Autodesk Inventor part; units mm, degrees
ref_plane "YZ Plane" through (0, 0, 0) normal (1, 0, 0) x (0, 1, 0)
ref_plane "XZ Plane" through (0, 0, 0) normal (0, 1, 0) x (-1, 0, 0)
ref_plane "XY Plane" through (0, 0, 0) normal (0, 0, 1) x (1, 0, 0)
sketch "スケッチ1" plane through (0, 0, 0) normal (0, 0, 1) x (1, 0, 0)
  line L0 (-29, -29) -> (29, -29)
  line L1 (29, -29) -> (29, 29)
  line L2 (29, 29) -> (-29, 29)
  line L3 (-29, 29) -> (-29, -29)
  line L4 (-29, -29) -> (29, 29) construction
  line L5 (29, -29) -> (-29, 29) construction
  point P0 (0, 0)
  dimension "d0" = 58
  dimension "d1" = 58
extrude "押し出し1" add sketch "スケッチ1" along normal blind 6
fillet "フィレット1" radius 5 4 edges at (-29, 29, 3) (29, 29, 3) (29, -29, 3) (-29, -29, 3)
sketch "スケッチ4" plane through (0, 0, 6) normal (0, 0, 1) x (1, 0, 0)
  arc A0 (-29, -24) -> (-24, -29) centre (-24, -24) ccw
  line L0 (-24, -29) -> (24, -29)
  arc A1 (24, -29) -> (29, -24) centre (24, -24) ccw
  line L1 (29, -24) -> (29, 24)
  arc A2 (29, 24) -> (24, 29) centre (24, 24) ccw
  line L2 (24, 29) -> (-24, 29)
  arc A3 (-24, 29) -> (-29, 24) centre (-24, 24) ccw
  line L3 (-29, 24) -> (-29, -24)
  line L4 (-27, -27) -> (27, -27)
  line L5 (27, -27) -> (27, 27)
  line L6 (27, 27) -> (-27, 27)
  line L7 (-27, 27) -> (-27, -27)
  line L8 (-27, -27) -> (27, 27) construction
  line L9 (27, -27) -> (-27, 27) construction
  line L10 (-24, -24) -> (24, -24) construction
  line L11 (24, -24) -> (24, 24) construction
  line L12 (24, 24) -> (-24, 24) construction
  line L13 (-24, 24) -> (-24, -24) construction
  line L14 (-24, -24) -> (24, 24) construction
  line L15 (24, -24) -> (-24, 24) construction
  line L16 (24, 29) -> (-24, 29)
  circle A4 centre (-24, 24) radius 5
  circle A5 centre (24, 24) radius 5
  arc A6 (24, -29) -> (29, -24) centre (24, -24) ccw
  circle A7 centre (24, -24) radius 5
  line L17 (-24, -29) -> (24, -29)
  circle A8 centre (-24, -24) radius 5
  line L18 (-29, 29) -> (-19, 29)
  line L19 (-19, 29) -> (-19, 19)
  line L20 (-19, 19) -> (-29, 19)
  line L21 (-29, 19) -> (-29, 29)
  line L22 (-29, 29) -> (-19, 19) construction
  line L23 (-19, 29) -> (-29, 19) construction
  line L24 (29, 29) -> (19, 29)
  line L25 (19, 29) -> (19, 19)
  line L26 (19, 19) -> (29, 19)
  line L27 (29, 19) -> (29, 29)
  line L28 (29, 29) -> (19, 19) construction
  line L29 (19, 29) -> (29, 19) construction
  line L30 (29, -29) -> (19, -29)
  line L31 (19, -29) -> (19, -19)
  line L32 (19, -19) -> (29, -19)
  line L33 (29, -19) -> (29, -29)
  line L34 (29, -29) -> (19, -19) construction
  line L35 (19, -29) -> (29, -19) construction
  line L36 (-29, -29) -> (-19, -29)
  line L37 (-19, -29) -> (-19, -19)
  line L38 (-19, -19) -> (-29, -19)
  line L39 (-29, -19) -> (-29, -29)
  line L40 (-29, -29) -> (-19, -19) construction
  line L41 (-19, -29) -> (-29, -19) construction
  point P0 (0, 0)
  point P1 (-20, -27)
  point P2 (20, -27)
  point P3 (27, -20)
  point P4 (27, 20)
  point P5 (20, 27)
  point P6 (-20, 27)
  point P7 (-27, 20)
  point P8 (-27, -20)
  point P9 (-19, -24)
  point P10 (-19, -27)
  point P11 (19, -27)
  point P12 (19, -24)
  point P13 (24, -19)
  point P14 (27, -19)
  point P15 (27, 19)
  point P16 (24, 19)
  point P17 (19, 24)
  point P18 (19, 27)
  point P19 (-19, 27)
  point P20 (-19, 24)
  point P21 (-24, 19)
  point P22 (-27, 19)
  point P23 (-27, -19)
  point P24 (-24, -19)
  dimension "d77" = 54
  dimension "d78" = 54
  dimension "d79" = 48
  dimension "d80" = 48
  dimension "d81" = 10
  dimension "d82" = 10
  dimension "d83" = 10
  dimension "d84" = 10
  dimension "d85" = 10
  dimension "d86" = 10
  dimension "d87" = 10
  dimension "d88" = 10
  dimension "d89" = 10
  dimension "d90" = 10
  dimension "d91" = 10
  dimension "d92" = 10
extrude "押し出し2" cut sketch "スケッチ4" against normal blind 4 contours L7 L20 L19 L6 L25 L26 L5 L32 L31 L4 L37 L38
sketch "スケッチ5" plane through (0, 0, 2) normal (0, 0, 1) x (1, 0, 0)
  circle A0 centre (0, 0) radius 16
  point P0 (-11.3137, 11.3137)
  point P1 (-11.3137, -11.3137)
  point P2 (11.3137, -11.3137)
  point P3 (11.3137, 11.3137)
  dimension "d18" = 32
  dimension "d21" = 360
  dimension "d58" = 0
hole "穴2" at (-11.3137, 11.3137, 2) at (-11.3137, -11.3137, 2) at (11.3137, -11.3137, 2) at (11.3137, 11.3137, 2) direction (0, 0, -1) diameter 4.5 depth 11.8 tip angle 118 counterbore diameter 8 counterbore depth 4
sketch "スケッチ6" plane through (0, 0, 2) normal (0, 0, 1) x (1, 0, 0)
  circle A0 centre (0, 0) radius 15
  point P0 (0, 15)
  point P1 (-15, 0)
  point P2 (0, -15)
  point P3 (15, 0)
  dimension "d30" = 30
  dimension "d33" = 360
  dimension "d59" = 0
hole "穴3" at (15, 0, 2) at (0, 15, 2) at (-15, 0, 2) direction (0, 0, -1) diameter 3.4 depth 11.8 tip angle 118
fillet "フィレット5" radius 3 8 edges at (-27, 19, 4) (-19, 27, 4) (19, 27, 4) (27, 19, 4) (27, -19, 4) (19, -27, 4) (-19, -27, 4) (-27, -19, 4)
sketch "スケッチ7" plane through (0, 0, 2) normal (0, 0, 1) x (1, 0, 0)
  circle A0 centre (0, 0) radius 10
  dimension "d42" = 20
extrude "押し出し3" cut sketch "スケッチ7" against normal through all
sketch "スケッチ8" plane through (0, 0, 6) normal (0, 0, 1) x (1, 0, 0)
  line L0 (24, -24) -> (-24, -24)
  line L1 (-24, -24) -> (-24, 24)
  line L2 (-24, 24) -> (24, 24)
  line L3 (24, 24) -> (24, -24)
  line L4 (24, -24) -> (-24, 24) construction
  line L5 (-24, -24) -> (24, 24) construction
  point P0 (0, 0)
  dimension "d45" = 48
  dimension "d46" = 48
hole "穴4" at (-24, 24, 6) at (-24, -24, 6) at (24, -24, 6) at (24, 24, 6) direction (0, 0, -1) diameter 3.4 depth 6 tip angle 118
sketch "スケッチ9" plane through (0, 0, 6) normal (0, 0, 1) x (1, 0, 0)
  line L0 (-20, -29) -> (20, -29)
  line L1 (20, -29) -> (20, -5)
  line L2 (20, -5) -> (-20, -5)
  line L3 (-20, -5) -> (-20, -29)
  line L4 (-20, -29) -> (20, -5) construction
  line L5 (20, -29) -> (-20, -5) construction
  line L6 (-24, -29) -> (24, -29)
  circle A0 centre (11.3137, -11.3137) radius 4
  line L7 (10, 5) -> (-10, 5)
  line L8 (-10, 5) -> (-10, -5)
  line L9 (-10, -5) -> (10, -5)
  line L10 (10, -5) -> (10, 5)
  line L11 (10, 5) -> (-10, -5) construction
  line L12 (-10, 5) -> (10, -5) construction
  circle A1 centre (0, 0) radius 10
  line L13 (-10, 0) -> (10, 0)
  point P0 (0, -17)
  point P1 (0, -17)
  point P2 (8.6603, -5)
  point P3 (-8.6603, -5)
  point P4 (-15, 0)
  dimension "d54" = 40
  dimension "d64" = 5
extrude "押し出し4" cut sketch "スケッチ9" against normal through all contours L3 L2 A1 L1 L0 | L8 A1 L2 | L2 A1 L10 | L2 A1 | A0
fillet "フィレット7" radius 5 2 edges at (-10, -5, 1) (10, -5, 1)
fillet "フィレット8" radius 2 2 edges at (-20, -5, 1) (20, -5, 1)
sketch "スケッチ11" plane through (0, 0, 0) normal (0, 0, -1) x (-1, 0, 0)
  circle A0 centre (24, 24) radius 1.7
  circle A1 centre (24, -24) radius 1.7
  circle A2 centre (-24, 24) radius 1.7
  circle A3 centre (-24, -24) radius 1.7
  line L0 (26.8, 25.6166) -> (26.8, 22.3834)
  line L1 (26.8, 22.3834) -> (24, 20.7668)
  line L2 (24, 20.7668) -> (21.2, 22.3834)
  line L3 (21.2, 22.3834) -> (21.2, 25.6166)
  line L4 (21.2, 25.6166) -> (24, 27.2332)
  line L5 (24, 27.2332) -> (26.8, 25.6166)
  line L6 (-24, 29) -> (24, 29)
  line L7 (21.2, -25.6166) -> (21.2, -22.3834)
  line L8 (21.2, -22.3834) -> (24, -20.7668)
  line L9 (24, -20.7668) -> (26.8, -22.3834)
  line L10 (26.8, -22.3834) -> (26.8, -25.6166)
  line L11 (26.8, -25.6166) -> (24, -27.2332)
  line L12 (24, -27.2332) -> (21.2, -25.6166)
  line L13 (-21.2, 25.6166) -> (-21.2, 22.3834)
  line L14 (-21.2, 22.3834) -> (-24, 20.7668)
  line L15 (-24, 20.7668) -> (-26.8, 22.3834)
  line L16 (-26.8, 22.3834) -> (-26.8, 25.6166)
  line L17 (-26.8, 25.6166) -> (-24, 27.2332)
  line L18 (-24, 27.2332) -> (-21.2, 25.6166)
  line L19 (24, -29) -> (20, -29)
  line L20 (-21.2, -22.3834) -> (-21.2, -25.6166)
  line L21 (-21.2, -25.6166) -> (-24, -27.2332)
  line L22 (-24, -27.2332) -> (-26.8, -25.6166)
  line L23 (-26.8, -25.6166) -> (-26.8, -22.3834)
  line L24 (-26.8, -22.3834) -> (-24, -20.7668)
  line L25 (-24, -20.7668) -> (-21.2, -22.3834)
  arc A4 (-29, -24) -> (-24, -29) centre (-24, -24) ccw
  line L26 (-20, -29) -> (-24, -29)
  line L27 (-29, -24) -> (-24, -29)
  point P0 (0, 0)
  point P1 (-25.8144, -26.1856)
  point P2 (-26.8, -25.2)
  dimension "d31" = 4
  dimension "d67" = 5.6
  dimension "d68" = 30
  dimension "d69" = 5.6
  dimension "d70" = 30
  dimension "d71" = 30
  dimension "d72" = 5.6
  dimension "d73" = 15
  dimension "d74" = 5.6
extrude "押し出し5" cut sketch "スケッチ11" against normal blind 4 contours A0 | A1 | A2 | A3 | L0 L1 L2 L3 L4 L5 | L7 L8 L9 L10 L11 L12 | L13 L14 L15 L16 L17 L18 | L20 L21 L22 L23 L24 L25
sketch "スケッチ12" plane through (0, 0, 6) normal (0, 0, 1) x (1, 0, 0)
  line L0 (-21, 25) -> (-3.9723, 25)
  line L1 (-3.9723, 25) -> (-3.9723, 27)
  line L2 (-3.9723, 27) -> (-21, 27)
  line L3 (-21, 27) -> (-21, 25)
  line L4 (-21, 25) -> (-3.9723, 27) construction
  line L5 (-3.9723, 25) -> (-21, 27) construction
  line L6 (24, 29) -> (-24, 29)
  line L7 (29, -24) -> (29, 24)
  line L8 (-29, 24) -> (-29, -24)
  line L9 (-19, 19) -> (-19, 24)
  line L10 (-19, 24) -> (-17.5063, 24)
  line L11 (-17.5063, 24) -> (-17.5063, 25)
  line L12 (-17.5063, 25) -> (-19, 25)
  line L13 (-19, 25) -> (-19, 24)
  point P0 (0, 0)
  point P1 (-12.4862, 26)
  point P2 (29, -19)
  dimension "d93" = 3
  dimension "d98" = 8
  dimension "d99" = 2
extrude "押し出し6" cut sketch "スケッチ12" against normal up to surface (4 mm away)
fillet "フィレット9" radius 4 2 edges at (-20, -19, 4) (20, -19, 4)
fillet "フィレット10" radius 5 2 edges at (19, 19, 4) (-19, 19, 4)
equation "\"d0\" = d1"
equation "\"d78\" = d77"
equation "\"d81\" = d89"
equation "\"d82\" = d89"
equation "\"d83\" = d90"
equation "\"d84\" = d90"
equation "\"d85\" = d92"
equation "\"d86\" = d92"
equation "\"d87\" = d91"
equation "\"d88\" = d91"
equation "\"d89\" = d90"
equation "\"d91\" = d89"
equation "\"d92\" = d91"
properties part number "base47" material "ABS プラスチック"
Input: part model. Units: mm. Frame: model coordinates. A direction names the side the tool comes from. Coordinates: 2 decimals unless noted, no trailing zeros. Write each loop counter-clockwise with the first axis right and the second up, starting at its lowest first coordinate (ties: lowest second). Pieces come first, ordered by that corner, then holes. Notation, with made-up numbers: (29.25, 57.25) -> (51.25, 57.25) arc R32 ccw to (51.25, 88.25) -> close; hole circle Ø5 at (-16.75, 46). An arc over 180 degrees is marked (long way). Answer as a JSON object with one key per item and string values.
1. Section B-B on x = -1. Return the cut outline in (y, z).
Result set:
{"outline": "(9.95, 0) -> (13.63, 0) -> (13.63, 2) -> (9.95, 2) -> close; (16.37, 0) -> (29, 0) -> (29, 6) -> (27, 6) -> (27, 2) -> (16.37, 2) -> close"}
2. Access query for faces 4 (the face through (21, 20, 4)), 5 (the face through (-11, -3, 1)), 6 (the face through (-22.7, -25.4, 4)), 7 (the face through (18.1, 26.14, 3.97)). Directions: +Z, -Z, +X, -X, +Y, -Y. A direction counts if a zero-diameter tool reaches every point of the face in a straight line with its end or side. Return the directions, or none.
Result set:
{"face 4": "+Z", "face 5": "+Z, -Z, -Y", "face 6": "-Z", "face 7": "+Z, -Y"}
3. Material intervals for line 1 (X direction, y = 0, z = 1.6); line 2 (X direction, y = -24, z = 5.1); line 3 (X direction, y = 6, z = 2.6), sorted ascending. Write a range as from..to.
Result set:
{"line 1": "x = -29..-16.7, -13.3..-10, 10..13.3, 16.7..29", "line 2": "x = -29..-25.7, -22.3..-20, 20..22.3, 25.7..29", "line 3": "x = -29..-27, 27..29"}
4. Section D-D on y = 12. Return the cut outline in (x, z).
Result set:
{"outline": "(-29, 0) -> (-15.25, 0) -> (-15.25, 2) -> (-27, 2) -> (-27, 6) -> (-29, 6) -> close; (-7.37, 0) -> (7.37, 0) -> (7.37, 2) -> (-7.37, 2) -> close; (15.25, 0) -> (29, 0) -> (29, 6) -> (27, 6) -> (27, 2) -> (15.25, 2) -> close"}
5. Section A-A on y = 20. Return the cut outline in (x, z).
Result set:
{"outline": "(-29, 0) -> (29, 0) -> (29, 6) -> (21, 6) -> (21, 2) -> (-21, 2) -> (-21, 6) -> (-29, 6) -> close"}
6. Section C-C on z = 3.2. Count the separate pieces of the cut face and the enclosed holes in it, then the cut area to 3 significant figures.
Result set:
{"separate pieces": "1", "enclosed holes": "4", "area": "466 mm2"}
7. Mould query, pull axis X, two halves, no side actions, for faces 1 (the face through (-22.62, 21.564, 1.972)), 2 (the face through (-2, 28, 6)), 3 (the face through (27, -28, 3)). Classes: released by +X, released by -X, zero draft, split by the parting line, or undercut.
Result set:
{"face 1": "undercut", "face 2": "zero draft", "face 3": "released by +X"}
8. First-contact query: P1, Ø3, axis at x = -11, z = 4.5, coming from the -Y side; P2, Ø0.5, axis at y = 24.5, z = 3.5, coming from the +X side; P3, Ø4.5, axis at x = 23.5, y = -23, coming from the -Z side; P4, Ø4.5, axis at x = 23.5, y = 24, coming from the -Z side. Flat tips, straight axial feed; report the tip coordinate or a pass-through.
Result set:
{"P1": "stops at y = 27", "P2": "stops at x = 28.99", "P3": "stops at z = 0", "P4": "stops at z = 4"}
